Work out the finished part from the listing and answer in its coordinate system (mm). A direction names the side the tool comes from. Round coordinates to 2 decimals unless told otherwise and drop trailing zeros. Write each loop counter-clockwise with the first axis right and the second up, starting at its lowest first coordinate (ties: lowest second). Pieces come first, ordered by that corner, then holes. Notation, with made-up numbers: (-4, 81.25) -> (15, 81.25) arc R30 ccw to (15, 106.25) -> close; hole circle Ø9 at (34.25, -6.75). An arc over 180 degrees is marked (long way). One line per item, written item: value.
```python
from build123d import *

# Parameters (mm, degrees)
SKETCH1_W           = 50
SKETCH1_H           = 50
BOSS_EXTRUDE1_DEPTH = 100
SKETCH2_R           = 9.9
BOSS_EXTRUDE2_DEPTH = 50
SKETCH3_R           = 10
CUT_EXTRUDE1_DEPTH  = 50


with BuildPart() as part:
    # Sketch1 → Boss-Extrude1 (new body)
    with BuildSketch(Plane.XY):
        with Locations((-25, 25)):
            Rectangle(SKETCH1_W, SKETCH1_H)
    extrude(amount=BOSS_EXTRUDE1_DEPTH)

    # Sketch2 → Boss-Extrude2 (add)
    with BuildSketch(Plane.ZY.offset(50)):
        with Locations(Location((75, 25, 0), (0, 0, 180))):
            Circle(SKETCH2_R)
    extrude(amount=BOSS_EXTRUDE2_DEPTH)

    # Sketch3 → Cut-Extrude1 (cut)
    with BuildSketch(Plane.XY.offset(100)):
        with Locations((-25, 25)):
            Circle(SKETCH3_R)
    extrude(amount=-CUT_EXTRUDE1_DEPTH, mode=Mode.SUBTRACT)


solid = part.part
```
(1) Find section A-A on z = 74.5. Give the vertices of the cut face in (x, y), plus the area to 3 significant figures.
Reported:
outline: (-100, 15.11) -> (-50, 15.11) -> (-50, 0) -> (0, 0) -> (0, 50) -> (-50, 50) -> (-50, 34.89) -> (-100, 34.89) -> close; hole circle Ø20 at (-25, 25)
area: 3,170 mm2
(2) Flat-ended cylindrical pins translate along their axes: pin 1 Ø12 at (x, y) = (-25, 25) entering from +Z; pin 2 Ø6 at (x, y) = (-71, 33.5) entering from -Z; pin 3 Ø15 at (y, z) = (22, 45.5) entering from -X. Find the tip coordinate at first contact, or state that the pin passes through.
Reported:
pin 1: stops at z = 50
pin 2: stops at z = 66.77
pin 3: stops at x = -50
(3) Find section D-D on z = 26. Give the vertices of the cut face in (x, y).
Reported:
outline: (-50, 0) -> (0, 0) -> (0, 50) -> (-50, 50) -> close
(4) For a pull along Y with two mould halves and no side action, classify faces 1 (the face through (-25, 25, 0)), 2 (the face through (-74.65, 28.792, 65.855)), 3 (the face through (-25, 25, 50)) as pulls with the +Y half, pulls with the -Y half, needs draft (parallel to the pull), parting line crosses it, or undercut.
Reported:
face 1: needs draft
face 2: parting line crosses it
face 3: undercut
(5) A tool of negligible diameter and unlimited length cuts with its end or side. For faces 4 (the face through (-15.46, 28, 75.35)), 5 (the face through (-100, 25, 75)), from which of +Z, -Z, +X, -X, +Y, -Y can it reach the whole face along a straight path? Write none if from no direction.
Reported:
face 4: +Z
face 5: +Z, -Z, -X, +Y, -Y
(6) Find section C-C on y = 29.5. Give the vertices of the cut face in (x, z), plus the area to 3 significant figures.
Reported:
outline: (-100, 66.18) -> (-50, 66.18) -> (-50, 0) -> (0, 0) -> (0, 100) -> (-16.07, 100) -> (-16.07, 50) -> (-33.93, 50) -> (-33.93, 100) -> (-50, 100) -> (-50, 83.82) -> (-100, 83.82) -> close
area: 4,990 mm2
(7) Find section B-B on x = -25. Give the vertices of the cut face in (y, z).
Reported:
outline: (0, 0) -> (50, 0) -> (50, 100) -> (35, 100) -> (35, 50) -> (15, 50) -> (15, 100) -> (0, 100) -> close
(8) Consider probe 1 along Y at (x, z) = (-25, 71); probe 2 along X at (y, z) = (40, 63); probe 3 along Z at (x, y) = (-81.5, 20). Determine where each line is inside the solid, lowest interval first.
Reported:
probe 1: y = 0 to 15, 35 to 50
probe 2: x = -50 to 0
probe 3: z = 66.46 to 83.54
